from build123d import *

# Parameters (mm, degrees)
F0_R     = 2
F0_W     = 13
F0_H     = 46.5
F0_W_2   = 15
F0_H_2   = 30
F1_DEPTH = 1


with BuildPart() as f1:
    # F0 (on Right) → F1 (new body)
    with BuildSketch(Plane.YZ):
        Polygon((21, 97.677421), (-5, 97.677421), (-5, -93.322579), (21, -93.322579), (21, 19.677421), (33.216004, 24.123683), (33.216004, 67.123683), (21, 71.569945), align=None)
        with Locations((8, -82.322579)):
            Circle(F0_R, mode=Mode.SUBTRACT)
        with Locations((8.5, -24.572579)):
            Rectangle(F0_W, F0_H, mode=Mode.SUBTRACT)
        with Locations((8, 14.677421)):
            Circle(F0_R, mode=Mode.SUBTRACT)
        with Locations((7.5, 45.677421)):
            Rectangle(F0_W_2, F0_H_2, mode=Mode.SUBTRACT)
        with Locations((8, 87.677421)):
            Circle(F0_R, mode=Mode.SUBTRACT)
    extrude(amount=F1_DEPTH)


solid = f1.part
For this review, take the finished solid that the model builds, in its own axes (mm). Coordinates: 2 decimals unless noted, no trailing zeros. Loops run counter-clockwise (first coordinate to the right, second up) from the corner with the lowest first, then second, coordinate; pieces in that order, holes last. Notation, with made-up numbers: (83, 45) -> (130, 45) arc R10 cw to (130, 61) -> close; hole circle Ø1 at (-12, -31). An arc over 180 degrees is marked (long way). Write each question's results on one line, items separated by ' | '.
Q1. Add section D-D, the plane z = 34. State the section outline as (x, y) points, then the cut area to 3 significant figures.
Taken from the geometry:
outline: (0, -5) -> (1, -5) -> (1, 0) -> (0, 0) -> close; (0, 15) -> (1, 15) -> (1, 33.22) -> (0, 33.22) -> close | area: 23.2 mm²
Q2. Add section B-B, the plane z = -8. State the section outline as (x, y) points.
Taken from the geometry:
outline: (0, -5) -> (1, -5) -> (1, 2) -> (0, 2) -> close; (0, 15) -> (1, 15) -> (1, 21) -> (0, 21) -> close
Q3. To check wall thickness, follow line 1 along Z through (x, y) = (0.75, 8); line 2 along Y through (x, z) = (0.4, 35); line 3 along Y through (x, z) = (0.25, -2). State the ranges of each line that lie inside material, in increasing order. Write a range as [from, to].
Taken from the geometry:
line 1: [-93.32, -84.32], [-80.32, -47.82], [-1.32, 12.68], [16.68, 30.68], [60.68, 85.68], [89.68, 97.68] | line 2: [-5, 0], [15, 33.22] | line 3: [-5, 2], [15, 21]
Q4. For pin 1 Ø0.5 at (x, z) = (0.5, -20) entering from +Y, flat-tipped, find the tip position at first contact; note if it passes through.
Taken from the geometry:
pin 1: y = 21
Q5. Mouldability with a two-part tool opening along Z and no side actions: class faces 1 (the cylindrical face through (0.493, 7.566, -84.275)), 2 (the flat face through (0.49, 27.02, 21.87)), 3 (the flat face through (0.493, 27.194, 69.316)) as +Z half, -Z half, draft (parallel to the pull), parting line (faces both ways), or undercut.
Taken from the geometry:
face 1: undercut | face 2: -Z half | face 3: +Z half
Q6. Add section A-A, the plane y = 8. State the section outline as (x, z) points.
Taken from the geometry:
outline: (0, -93.32) -> (1, -93.32) -> (1, -84.32) -> (0, -84.32) -> close; (0, -80.32) -> (1, -80.32) -> (1, -47.82) -> (0, -47.82) -> close; (0, -1.32) -> (1, -1.32) -> (1, 12.68) -> (0, 12.68) -> close; (0, 16.68) -> (1, 16.68) -> (1, 30.68) -> (0, 30.68) -> close; (0, 60.68) -> (1, 60.68) -> (1, 85.68) -> (0, 85.68) -> close; (0, 89.68) -> (1, 89.68) -> (1, 97.68) -> (0, 97.68) -> close
Q7. Add section C-C, the plane x = 0.65. State the section outline as (y, z) points.
Taken from the geometry:
outline: (-5, -93.32) -> (21, -93.32) -> (21, 19.68) -> (33.22, 24.12) -> (33.22, 67.12) -> (21, 71.57) -> (21, 97.68) -> (-5, 97.68) -> close; hole (0, 30.68) -> (15, 30.68) -> (15, 60.68) -> (0, 60.68) -> close; hole (2, -47.82) -> (15, -47.82) -> (15, -1.32) -> (2, -1.32) -> close; hole circle Ø4 at (8, -82.32); hole circle Ø4 at (8, 14.68); hole circle Ø4 at (8, 87.68)
